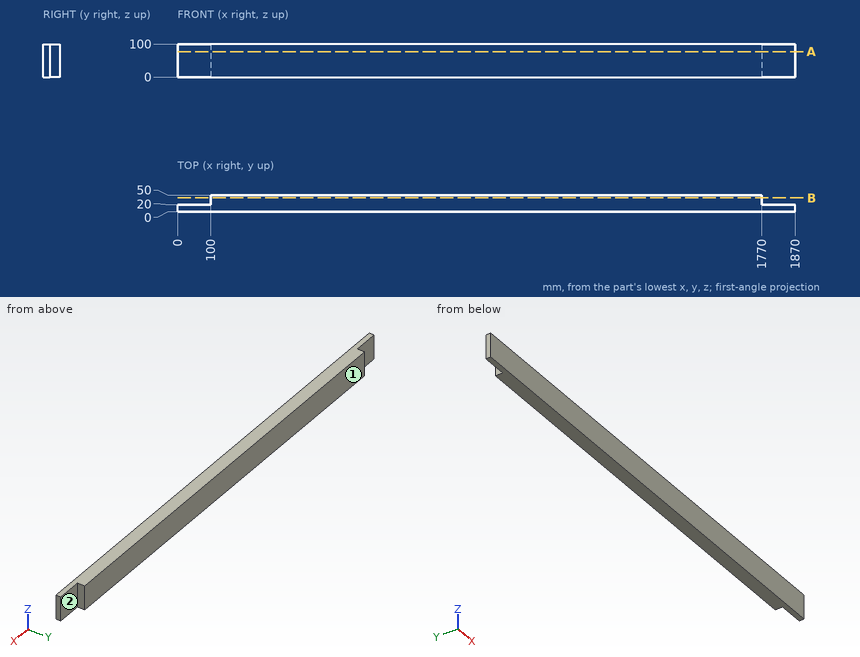
Geometry check sheet. Reference: drawing and pictorial views, mm from the part's lowest x, y, z. A direction names the side the tool comes from. Coordinates: 2 decimals unless noted, no trailing zeros. Write each loop counter-clockwise with the first axis right and the second up, starting at its lowest first coordinate (ties: lowest second). Pieces come first, ordered by that corner, then holes. Notation, with made-up numbers: (12, 53) - (60, 53) arc R31 ccw to (60, 91) - close; hole circle Ø8 at (-21.5, -13). An arc over 180 degrees is marked (long way). One line per question, with ' | ' between items. Start each with the question number.
1. Gauge pin test, flat end, axial feed: P1, Ø24, axis at y = 42, z = 44, coming from the -X side. Record the tip position at first contact, or that the pin passes through.
2. Material ranges on line 1 along X through (y, z) = (48, 41.5), recorded low to high.
3. Section check B-B (y = 41). Enter the section's corners in (x, z).
4. Section check A-A (z = 77). Enter the section's corners in (x, y), plus the area to 3 significant figures.
5. Access from +Z, -Z, +X, -X, +Y, -Y to the whole of each face (thin tool, end or side, straight path). Record for the marked faces 1 and 2.
Computed values:
1) P1: x = 100
2) line 1: 100 to 1770
3) outline: (100, 0) - (1770, 0) - (1770, 100) - (100, 100) - close
4) outline: (0, 0) - (1870, 0) - (1870, 20) - (1770, 20) - (1770, 50) - (100, 50) - (100, 20) - (0, 20) - close | area: 87,500 mm²
5) face 1: +Z, -Z, +X, -X, +Y | face 2: +Z, -Z, +X, +Y
